from build123d import *

# Parameters (mm, degrees)
PAD114_DEPTH    = 3.6
SKETCH245_W     = 199.954956
SKETCH245_H     = 336.690071
POCKET129_DEPTH = 50
POCKET130_DEPTH = 300
SKETCH247_R     = 4.05
POCKET131_DEPTH = 5
SKETCH248_R     = 0.8
POCKET132_DEPTH = 10
SKETCH249_R     = 1.75
POCKET133_DEPTH = 4.5


with BuildPart() as part:
    # Sketch244 → Pad114 (new body)
    with BuildSketch(Plane.XZ):
        with BuildLine():
            add(Edge.make_bspline(
                [(299.999063, 0.026825), (299.662766, 0.037193), (298.339429, 0.190401), (295.439956, 0.589669), (290.775356, 1.337839), (284.500044, 2.393262), (276.735212, 3.66473), (267.577355, 5.083019), (257.136483, 6.653879), (245.549215, 8.381993), (232.975291, 10.222771), (219.590016, 12.153256), (205.573823, 14.115503), (191.111579, 16.055183), (176.381713, 17.897983), (161.544489, 19.553409), (146.739309, 20.940939), (132.087536, 21.99009), (117.705275, 22.664279), (103.703346, 22.961168), (90.192549, 22.858072), (77.284675, 22.375726), (65.094168, 21.544938), (53.730431, 20.369385), (43.29002, 18.857963), (33.852484, 17.043697), (25.485501, 14.967735), (18.252292, 12.67281), (12.179436, 10.224412), (7.338355, 7.689021), (3.623023, 5.152403), (1.3546, 2.748114), (-0.314638, 0.590402), (0.575789, -1.804065), (3.482069, -2.72942), (7.386052, -3.91761), (13.030922, -4.754284), (20.096342, -5.463024), (28.645402, -5.933379), (38.56853, -6.201185), (49.790194, -6.284208), (62.196701, -6.193111), (75.660953, -5.967607), (90.034637, -5.629522), (105.153445, -5.226063), (120.83724, -4.775199), (136.895942, -4.296045), (153.13493, -3.818601), (169.356828, -3.345106), (185.36574, -2.889379), (200.968742, -2.465331), (215.974941, -2.074889), (230.201502, -1.715375), (243.47905, -1.394255), (255.639348, -1.103787), (266.55871, -0.849968), (276.034544, -0.603524), (284.209012, -0.340437), (290.324953, -0.117215), (295.955653, 0.018504), (297.364702, 0.013759), (300.343856, 0.01512), (300.000055, 0.026794), (299.999063, 0.026825)],
                knots=[0, 0, 0, 0, 1.017748, 3.99659, 8.779341, 15.189917, 23.087031, 32.383824, 42.990765, 54.76218, 67.530065, 81.114584, 95.333435, 109.988542, 124.889458, 139.866624, 154.774633, 169.496697, 183.930349, 197.964304, 211.506735, 224.45797, 236.709214, 248.156653, 258.723012, 268.346769, 276.97692, 284.567784, 291.102108, 296.573756, 300.992679, 304.39163, 306.761357, 308.43213, 311.131254, 315.298227, 320.951765, 328.080828, 336.654655, 346.609821, 357.866231, 370.316475, 383.83025, 398.264023, 413.449345, 429.202773, 445.334827, 461.646891, 477.940787, 494.021253, 509.693044, 524.767168, 539.054704, 552.387642, 564.607107, 575.560217, 585.109622, 593.180747, 599.700326, 604.53767, 607.540683, 608.560842, 608.563842, 608.563842, 608.563842, 608.563842], degree=3))
        make_face()
    extrude(amount=PAD114_DEPTH)

    # Sketch245 → Pocket129 (cut, symmetric)
    with BuildSketch(Plane.XY):
        with Locations((301.477478, -150.975887)):
            Rectangle(SKETCH245_W, SKETCH245_H)
    extrude(amount=POCKET129_DEPTH, both=True, mode=Mode.SUBTRACT)

    # Sketch246 (on Face4 of Pocket129) → Pocket130 (cut)
    with BuildSketch(Plane.XZ.offset(3.6)):
        with BuildLine():
            ThreePointArc((202, 14.6), (193.4, 6), (202, -2.6))
            Line((213.747525, -30.946017), (202, -2.6))
            Line((-22.89874, -30.946017), (213.747525, -30.946017))
            Line((-27.727513, 31.780215), (-22.89874, -30.946017))
            Line((188.968875, 46.453211), (-27.727513, 31.780215))
            Line((202, 14.6), (188.968875, 46.453211))
        make_face()
    extrude(amount=-POCKET130_DEPTH, mode=Mode.SUBTRACT)

    # Sketch247 (on Face4 of Pocket130) → Pocket131 (cut)
    with BuildSketch(Plane.XZ.offset(3.6)):
        with Locations((202, 6)):
            Circle(SKETCH247_R)
    extrude(amount=-POCKET131_DEPTH, mode=Mode.SUBTRACT)

    # Sketch248 (on Face7 of Pocket131) → Pocket132 (cut)
    with BuildSketch(Plane(origin=(201.5, 0, 0), x_dir=(0, 0, 1), z_dir=(1, 0, 0))):
        with Locations((12.3, 1.8)):
            Circle(SKETCH248_R)
        with Locations((-0.3, 1.8)):
            Circle(SKETCH248_R)
    extrude(amount=-POCKET132_DEPTH, mode=Mode.SUBTRACT)

    # Sketch249 (on DatumPlane) → Pocket133 (cut)
    with BuildSketch(Plane(origin=(193.5, 0, 0), x_dir=(0, 0, 1), z_dir=(1, 0, 0))):
        with Locations((12.3, 1.8)):
            Circle(SKETCH249_R)
        with Locations((-0.3, 1.8)):
            Circle(SKETCH249_R)
    extrude(amount=POCKET133_DEPTH, mode=Mode.SUBTRACT)


with BuildPart() as part_1:
    # Body047 placement: moved
    add(part.part.moved(Location((0, -609, 0))))


solid = part_1.part
The listing builds one solid part. Answer for the finished solid, in the listing's coordinates (mm). A direction names the side the tool comes from. Coordinates: 2 decimals unless noted, no trailing zeros. Loops run counter-clockwise (first coordinate to the right, second up) from the corner with the lowest first, then second, coordinate; pieces in that order, holes last.
1) Determine the mould class of faces 1 (the face through (197, -609, 6)), 2 (the face through (199.774, -611.593, -0.404)), 3 (the face through (201.5, -612, 12)) for opening direction Y: pulls with the +Y half, pulls with the -Y half, needs draft (parallel to the pull), parting line crosses it, or undercut.
2) Find the intervals of material crossed by L1, parallel to Z at x = 200.3, y = -610.8; L2, parallel to Z at x = 198.95, y = -610.8; L3, parallel to Y at x = 198.85, z = -0.3, in increasing order.
3) Find section C-C on y = -610.8. Give the number of separate pieces and of enclosed holes in the cut face, then the cut area to 3 significant figures.
4) Find section B-B on z = -0.3. Write down the section's boundary in (x, y), then the cut area to 3 significant figures.
5) Find section D-D on x = 196.5. Write down the section's boundary in (y, z).
6) A tool of negligible diameter and unlimited length cuts with its end or side. For faces 4 (the face through (198, -611, 1)), 5 (the face through (193.424, -610.825, 6.647)), from which of +Z, -Z, +X, -X, +Y, -Y can it reach the whole face along a straight path? Write none if from no direction.
7) Flat-ended cylindrical pins translate along their axes: pin 1 Ø0.9 at (y, z) = (-610.5, 0) entering from -X; pin 2 Ø1 at (y, z) = (-611, 7) entering from -X. Find the tip coordinate at first contact, or state that the pin passes through.
8) Find section A-A on x = 200. Write down the section's boundary in (y, z), then the cut area to 3 significant figures.
Values:
1. face 1: pulls with the +Y half
1. face 2: undercut
1. face 3: needs draft
2. L1: z = -2.43 to -1.1, 0.5 to 2.32, 9.68 to 11.5, 13.1 to 14.43
2. L2: z = -2.04 to -1.1, 0.5 to 3.34, 8.66 to 11.5, 13.1 to 14.04
2. L3: y = -612.6 to -611.6, -610 to -609
3. separate pieces: 3
3. enclosed holes: 0
3. area: 62.7 mm2
4. outline: (196.15, -612.6) - (201.5, -612.6) - (201.5, -611.6) - (198, -611.6) - (198, -612.55) - (196.15, -612.55) - close; (196.15, -609.05) - (198, -609.05) - (198, -610) - (201.5, -610) - (201.5, -609) - (196.15, -609) - close
4. area: 7.19 mm2
5. outline: (-612.6, -0.61) - (-612.52, -0.61) arc R1.75 cw (long way) to (-609.08, -0.61) - (-609, -0.61) - (-609, 12.61) - (-609.08, 12.61) arc R1.75 cw (long way) to (-612.52, 12.61) - (-612.6, 12.61) - close
6. face 4: -X
6. face 5: -X, +Y, -Y
7. pin 1: stops at x = 198
7. pin 2: stops at x = 193.41
8. outline: (-612.6, -2.36) - (-609, -2.36) - (-609, 2.48) - (-612.6, 2.48) - close; (-612.6, 9.52) - (-609, 9.52) - (-609, 14.36) - (-612.6, 14.36) - close; hole circle Ø1.6 at (-610.8, -0.3); hole circle Ø1.6 at (-610.8, 12.3)
8. area: 30.8 mm2
